Read the model definition and answer for the solid it produces. Units are mm, in the model's axes. Coordinates: 2 decimals unless noted, no trailing zeros. Loops run counter-clockwise (first coordinate to the right, second up) from the corner with the lowest first, then second, coordinate; pieces in that order, holes last. Notation, with made-up numbers: (-9.75, -12.5) -> (-1.75, -12.5) arc R23 cw to (-1.75, 1.5) -> close; hole circle Ø2 at (47.5, -34.5). An arc over 180 degrees is marked (long way). Answer as CSV lines item,"result".
```python
from build123d import *

# Parameters (mm, degrees)
ESQUISSE1_W        = 173
ESQUISSE1_H        = 273
ESQUISSE1_R        = 1.5
ESQUISSE1_W_2      = 52
ESQUISSE1_H_2      = 28
ESQUISSE1_W_3      = 81
ESQUISSE1_H_3      = 76
BOSS_EXTRU_1_DEPTH = 4
D_GAGEMENT_M31_D   = 3.4
CONG_1_R           = 3


with BuildPart() as part:
    # Esquisse1 → Boss.-Extru.1 (new body)
    with BuildSketch(Plane.XY):
        with Locations((86.5, 136.5)):
            Rectangle(ESQUISSE1_W, ESQUISSE1_H)
        with Locations((15, 236.5)):
            Circle(ESQUISSE1_R, mode=Mode.SUBTRACT)
        with Locations((165.38, 236.5)):
            Circle(ESQUISSE1_R, mode=Mode.SUBTRACT)
        with Locations((15, 70.5)):
            Circle(ESQUISSE1_R, mode=Mode.SUBTRACT)
        with Locations((100, 46)):
            Rectangle(ESQUISSE1_W_2, ESQUISSE1_H_2, mode=Mode.SUBTRACT)
        with Locations((74.5, 182)):
            Rectangle(ESQUISSE1_W_3, ESQUISSE1_H_3, mode=Mode.SUBTRACT)
    extrude(amount=BOSS_EXTRU_1_DEPTH)

    # Dégagement M31 (through all)
    with Locations(Plane.XY.offset(4)):
        with Locations((15, 236.5), (15, 70.5), (165.38, 236.5)):
            Hole(D_GAGEMENT_M31_D / 2)

    # Congé1
    cong_1_edges = [part.edges().sort_by_distance(p)[0] for p in [
        (74, 60, 2),
        (74, 32, 2),
        (126, 32, 2),
        (126, 60, 2),
        (34, 220, 2),
        (34, 144, 2),
        (115, 144, 2),
        (115, 220, 2),
        (0, 273, 2),
        (173, 273, 2),
        (173, 0, 2),
        (0, 0, 2),
    ]]
    fillet(cong_1_edges, radius=CONG_1_R)


solid = part.part
```
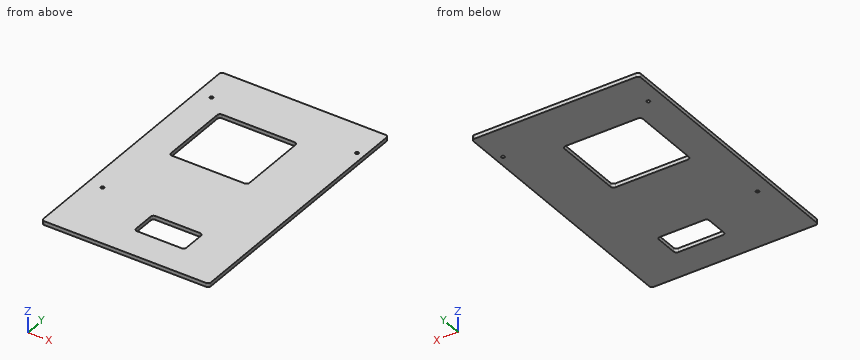
Q1. A cutting plane is placed at A-A, the plane x = 89. Write down the section's boundary in (y, z), and give its area (3 significant figures).
Results:
outline,"(0, 0) -> (32, 0) -> (32, 4) -> (0, 4) -> close; (60, 0) -> (144, 0) -> (144, 4) -> (60, 4) -> close; (220, 0) -> (273, 0) -> (273, 4) -> (220, 4) -> close"
area,"676 mm²"
Q2. Given pin 1 Ø3 at (x, y) = (15, 70.5) entering from +Z, flat-ended and moving along its own axis, determine where the tip first touches the part or whether it passes through.
Results:
pin 1,"passes through"
Q3. Find the intervals of material crossed by probe 1 along X at (y, z) = (236.5, 1); probe 2 along Y at (x, z) = (15, 2.7); probe 3 along Y at (x, z) = (165.38, 2.2), in increasing order. Write a range as [from, to].
Results:
probe 1,"x = [0, 13.3], [16.7, 163.68], [167.08, 173]"
probe 2,"y = [0, 68.8], [72.2, 234.8], [238.2, 273]"
probe 3,"y = [0, 234.8], [238.2, 273]"
Q4. A cutting plane is placed at C-C, the plane y = 180. Write down the section's boundary in (x, z).
Results:
outline,"(0, 0) -> (34, 0) -> (34, 4) -> (0, 4) -> close; (115, 0) -> (173, 0) -> (173, 4) -> (115, 4) -> close"
Q5. A cutting plane is placed at B-B, the plane z = 3.1. Write down the section's boundary in (x, y).
Results:
outline,"(0, 3) arc R3 ccw to (3, 0) -> (170, 0) arc R3 ccw to (173, 3) -> (173, 270) arc R3 ccw to (170, 273) -> (3, 273) arc R3 ccw to (0, 270) -> close; hole circle Ø3.4 at (15, 70.5); hole circle Ø3.4 at (15, 236.5); hole (34, 147) arc R3 ccw to (37, 144) -> (112, 144) arc R3 ccw to (115, 147) -> (115, 217) arc R3 ccw to (112, 220) -> (37, 220) arc R3 ccw to (34, 217) -> close; hole (74, 35) arc R3 ccw to (77, 32) -> (123, 32) arc R3 ccw to (126, 35) -> (126, 57) arc R3 ccw to (123, 60) -> (77, 60) arc R3 ccw to (74, 57) -> close; hole circle Ø3.4 at (165.38, 236.5)"
